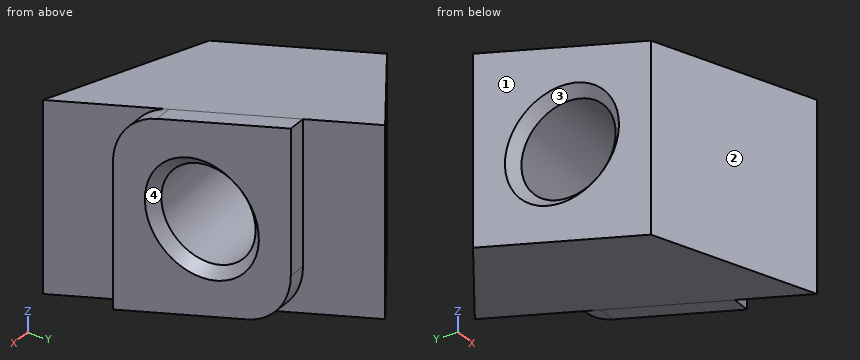
from build123d import *

# Parameters (mm, degrees)
EXTRUDE1_DEPTH = 0.8
EXTRUDE2_DEPTH = 5.5
DRAFT1_ANGLE   = -33.206570315
DRAFT2_ANGLE   = -33.206570315
HOLEWZD1_D     = 4.134
HOLEWZD1_DEPTH = 6.300025
CHAMFER1_SIZE  = 0.433


with BuildPart() as part:
    # Sketch1 → Extrude1 (new body)
    with BuildSketch(Plane(origin=(0, 0, 0), x_dir=(0, 0, -1), z_dir=(1, 0, 0))):
        with BuildLine():
            Line((1.101052702, 3.9), (-5.186106572, 3.9))
            Line((-5.186106572, 3.9), (-3.612459851, -1.972929517))
            ThreePointArc((-3.612459851, -1.972929517), (-2.683832418, -3.362718685), (-1.101052702, -3.9))
            Line((-1.101052702, -3.9), (5.186106572, -3.9))
            Line((5.186106572, -3.9), (3.612459851, 1.972929517))
            ThreePointArc((3.612459851, 1.972929517), (2.683832418, 3.362718685), (1.101052702, 3.9))
        make_face()
    extrude(amount=-EXTRUDE1_DEPTH)

    # Sketch2 → Extrude2 (add)
    with BuildSketch(Plane.ZY.offset(0.8)):
        with BuildLine():
            Line((2.131485778, -7.5), (-6.150723665, -7.5))
            add(Edge.make_bspline(
                [(-2.131485778, 7.5), (-3.471231741, 2.5), (-4.810977703, -2.5), (-6.150723665, -7.5)],
                knots=[0, 0, 0, 0, 1, 1, 1, 1], degree=3))
            Line((-2.131485778, 7.5), (6.150723665, 7.5))
            add(Edge.make_bspline(
                [(2.131485778, -7.5), (3.471231741, -2.5), (4.810977703, 2.5), (6.150723665, 7.5)],
                knots=[0, 0, 0, 0, 1, 1, 1, 1], degree=3))
        make_face()
    extrude(amount=EXTRUDE2_DEPTH)

    # Draft1
    draft1_faces = [part.faces().sort_by_distance(p)[0] for p in [
        (-3.55, 7.5, 2.009618943),
    ]]
    draft(draft1_faces, Plane(origin=(-0.8, 0, 4.141104722), x_dir=(0, 0, 1), z_dir=(1, 0, 0)), DRAFT1_ANGLE)

    # Draft2
    draft2_faces = [part.faces().sort_by_distance(p)[0] for p in [
        (-3.55, -7.5, -2.009618943),
    ]]
    draft(draft2_faces, Plane(origin=(-0.8, 0, 4.141104722), x_dir=(0, 0, 1), z_dir=(1, 0, 0)), DRAFT2_ANGLE)

    # HoleWzd1
    with Locations(Plane.ZY.offset(6.3)):
        with Locations((0, 0)):
            Hole(HOLEWZD1_D / 2, depth=HOLEWZD1_DEPTH)

    # Chamfer1
    chamfer1_edges = [part.edges().sort_by_distance(p)[0] for p in [
        (0, 0, 2.067),
        (-6.3, 0, 2.067),
    ]]
    chamfer(chamfer1_edges, length=CHAMFER1_SIZE)


solid = part.part
Design review of the part built by this model. Coordinates are the model's own, in mm. Face numbers are marked on the shaded views. Give positions to 0.01 mm unless a question says otherwise; leave off trailing zeros. Write each loop counter-clockwise with the first axis right and the second up, starting at its lowest first coordinate (ties: lowest second). Pieces come first, ordered by that corner, then holes. Notation, with made-up numbers: M 68.25,38 L 85.25,38 A15 cw 85.25,42 Z; hole C 14.25,4.5 d2. An arc over 180 degrees is marked long. Return JSON: item names as keys, results as strings. Group by question number.
Item 1: Take a section at B-B (x = -0.25). Give the boundary of the cut face in (y, z).
Item 2: Take a section at A-A (z = 0). Give the boundary of the cut face in (x, y), plus the area to 3 significant figures.
Item 3: Clearance check with flat-ended pins moving along their axes: pin 1 Ø1 at (x, z) = (-4, 1) entering from -Y; pin 2 Ø1 at (x, y) = (-1, 1.5) entering from -Z; pin 3 Ø0.9 at (x, z) = (-0.5, -1) entering from -Y; pin 4 Ø6.5 at (y, z) = (0, 0) entering from +X. State where each tip first meets the part, or that it passes through.
Item 4: The part is to be moulded in two halves that separate along Y. For the marked faces 1, 2, 3 and 4, say which applies: pulls with the +Y half, pulls with the -Y half, needs draft (parallel to the pull), parting line crosses it, or undercut.
Item 5: Wall thickness on line 1 along Y through (x, z) = (-6, -2); line 2 along Y through (x, z) = (-3, -0.25); line 3 along Y through (x, z) = (-5, -2.25): over which ranges is each line inside the solid? List them lowest first.
Return value:
{
 "1": {"outline": "M -3.9,-5.19 L 1.97,-3.61 A2.6 ccw 3.9,-1.1 L 3.9,5.19 L -1.97,3.61 A2.6 ccw -3.9,1.1 Z; hole C 0,0 d4.5"},
 "2": {"outline": "M -6.3,-3.9 L -0.8,-7.5 L -0.8,-3.9 L 0,-3.9 L 0,-2.5 L -0.43,-2.07 L -5.87,-2.07 L -6.3,-2.5 Z; M -6.3,2.5 L -5.87,2.07 L -0.43,2.07 L 0,2.5 L 0,3.9 L -0.8,3.9 L -0.8,7.5 L -6.3,3.9 Z", "area": "42.5 mm2"},
 "3": {"pin 1": "stops at y = -5.73", "pin 2": "stops at z = -3.87", "pin 3": "stops at y = -7.5", "pin 4": "stops at x = 0"},
 "4": {"face 1": "needs draft", "face 2": "pulls with the -Y half", "face 3": "undercut", "face 4": "undercut"},
 "5": {"line 1": "y = -4.1 to -0.92, 0.92 to 4.1", "line 2": "y = -6.06 to -2.05, 2.05 to 6.06", "line 3": "y = -4.75 to 4.75"}
}
